Could you check a few things on this model? Use its own coordinates, in mm. A direction names the side the tool comes from. Give positions to 0.01 mm unless a question says otherwise; leave off trailing zeros. Loops run counter-clockwise (first coordinate to the right, second up) from the corner with the lowest first, then second, coordinate; pieces in that order, holes last. Notation, with made-up numbers: (58.25, 18) -> (114.25, 18) arc R17 cw to (114.25, 23) -> close; hole circle Ø2 at (67.25, 86). An arc over 180 degrees is marked (long way). Write each question's results on one line, items separated by ' | '. Start each with the question number.
Q1. We'd pull the mould along Y, two halves only. Please class faces 1 (the face through (14.5, -3, 5)), 2 (the face through (-16, -1, 5)), 3 (the face through (0, 4, -3)), 4 (the face through (17.5, -0.5, 4.9)): released by +Y, released by -Y, zero draft, split by the parting line, or undercut.
Q2. If we section it at C-C, the plane z = 12: List the corners of the cut face in (x, y) for me.
Q3. If we section it at B-B, the plane x = 3: List the corners of the cut face in (y, z) for me.
Q4. If we section it at D-D, the plane x = -11: List the corners of the cut face in (y, z) for me.
Q5. If I drill on line 1 along Z through (x, y) = (3, 4.65); line 2 along X through (y, z) = (5.7, 12.5); line 3 along Y through (x, z) = (-12.5, 9.25), over which ranges is the centre line in solid material (lowest first)?
Q6. Which directions (+Z, -Z, +X, -X, +Y, -Y) give clear straight access to the entire face, cutting with the end or side of a thin tool? Please do faces 5 (the face through (16, -1, 5)), 6 (the face through (0, 1, 0)), 7 (the face through (0, 1, 10)).
Q7. Will these pins go through, and if not, where does the flat tip stop? P1, Ø0.9, axis at x = -15.5, z = 6, coming from the +Y side; P2, Ø8, axis at x = -6.5, z = 3.5, coming from the -Y side; P3, Ø1, axis at y = 5.5, z = 9, coming from the +X side; P4, Ø2.5, axis at y = 5, z = 4.5, coming from the -X side.
Q8. If we section it at A-A, the plane y = -3.75: List the corners of the cut face in (x, z) for me.
from build123d import *

# Parameters (mm, degrees)
BOSS_EXTRUDE1_DEPTH = 10
SKETCH3_W           = 30
SKETCH3_H           = 22
BOSS_EXTRUDE2_DEPTH = 3
SKETCH4_R           = 1.5
CUT_EXTRUDE1_DEPTH  = 5


with BuildPart() as part:
    # Sketch2 → Boss-Extrude1 (new body)
    with BuildSketch(Plane.XY):
        Polygon((-17.5, 0), (-17.5, -1), (-14.5, -1), (-14.5, -5), (-22.5, -5), (-22.5, 0), (-22.5, 4), (22.5, 4), (22.5, -5), (14.5, -5), (14.5, -1), (17.5, -1), (17.5, 0), align=None)
    extrude(amount=BOSS_EXTRUDE1_DEPTH)

    # Sketch3 → Boss-Extrude2 (add)
    with BuildSketch(Plane(origin=(0, 4, 0), x_dir=(1, 0, 0), z_dir=(0, 1, 0))):
        with Locations((0, -5)):
            Rectangle(SKETCH3_W, SKETCH3_H)
    extrude(amount=BOSS_EXTRUDE2_DEPTH)

    # Sketch4 → Cut-Extrude1 (cut)
    with BuildSketch(Plane(origin=(0, 7, 0), x_dir=(1, 0, 0), z_dir=(0, 1, 0))):
        with Locations((3, 2.5)):
            Circle(SKETCH4_R)
        with Locations((3, -12.5)):
            Circle(SKETCH4_R)
    extrude(amount=-CUT_EXTRUDE1_DEPTH, mode=Mode.SUBTRACT)


solid = part.part
Final values:
1) face 1: zero draft | face 2: undercut | face 3: released by -Y | face 4: undercut
2) outline: (-15, 4) -> (1.59, 4) -> (1.59, 7) -> (-15, 7) -> close; (4.41, 4) -> (15, 4) -> (15, 7) -> (4.41, 7) -> close
3) outline: (0, 0) -> (4, 0) -> (4, -1) -> (7, -1) -> (7, 11) -> (4, 11) -> (4, 10) -> (0, 10) -> close; (4, -6) -> (7, -6) -> (7, -4) -> (4, -4) -> close; (4, 14) -> (7, 14) -> (7, 16) -> (4, 16) -> close
4) outline: (0, 0) -> (4, 0) -> (4, -6) -> (7, -6) -> (7, 16) -> (4, 16) -> (4, 10) -> (0, 10) -> close
5) line 1: z = -6 to -4, -1 to 11, 14 to 16 | line 2: x = -15 to 1.5, 4.5 to 15 | line 3: y = 0 to 7
6) face 5: +Z, -Z | face 6: -Z, +X, -X, -Y | face 7: +Z, +X, -X, -Y
7) P1: stops at y = 4 | P2: stops at y = 0 | P3: stops at x = 15 | P4: stops at x = -22.5
8) outline: (-22.5, 0) -> (-14.5, 0) -> (-14.5, 10) -> (-22.5, 10) -> close; (14.5, 0) -> (22.5, 0) -> (22.5, 10) -> (14.5, 10) -> close
